```python
from build123d import *

# Parameters (mm, degrees)
BOSS_EXTRUDE1_DEPTH = 2.5
SKETCH2_R           = 1.2
CUT_EXTRUDE1_DEPTH  = 14.44432966


with BuildPart() as part:
    # Sketch1 → Boss-Extrude1 (new, symmetric)
    with BuildSketch(Plane.XY):
        with BuildLine():
            Line((5, 0), (11.5, 0))
            Line((11.5, 0), (11.5, -1.5))
            Line((11.5, -1.5), (6.32455532, -1.5))
            ThreePointArc((6.32455532, -1.5), (0, -6.5), (-6.32455532, -1.5))
            Line((-6.32455532, -1.5), (-11.5, -1.5))
            Line((-11.5, -1.5), (-11.5, 0))
            Line((-11.5, 0), (-5, 0))
            ThreePointArc((-5, 0), (0, -5), (5, 0))
        make_face()
    extrude(amount=BOSS_EXTRUDE1_DEPTH, both=True)

    # Sketch2 → Cut-Extrude1 (cut, through all)
    with BuildSketch(Plane(origin=(0, 0, 0), x_dir=(1, 0, 0), z_dir=(0, 1, 0))):
        with Locations(Location((-9, 0, 0), (0, 0, 270))):
            Circle(SKETCH2_R)
        with Locations(Location((9, 0, 0), (0, 0, 180))):
            Circle(SKETCH2_R)
    extrude(amount=-CUT_EXTRUDE1_DEPTH, mode=Mode.SUBTRACT)


solid = part.part
```
Design review of the part built by this model. Coordinates are the model's own, in mm. A direction names the side the tool comes from. Round coordinates to 2 decimals unless told otherwise and drop trailing zeros. Order: outer loops, then holes, each group sorted by start corner. A loop starts at its lowest first (then second) coordinate and runs counter-clockwise, first axis right, second up. Notation, with made-up numbers: (36, 10) - (61, 10) arc R23 ccw to (61, 32) - close; hole circle Ø6 at (42, -3.5). An arc over 180 degrees is marked (long way). Return JSON: item names as keys, results as strings.
Q1. Consider section D-D on y = -3.75. Write out the cut boundary in (x, z), plus the area to 3 significant figures.
Computed values:
{"outline": "(-5.31, -2.5) - (-3.31, -2.5) - (-3.31, 2.5) - (-5.31, 2.5) - close; (3.31, -2.5) - (5.31, -2.5) - (5.31, 2.5) - (3.31, 2.5) - close", "area": "20.0 mm2"}
Q2. For pin 1 Ø3 at (x, z) = (-2.5, 1.5) entering from +Y; pin 2 Ø2.5 at (x, z) = (-8, 1) entering from -Y, all flat-tipped, find the tip position at first contact; note any pin that passes through.
Computed values:
{"pin 1": "stops at y = -3", "pin 2": "stops at y = -1.5"}
Q3. Consider section C-C on z = 0. Write out the cut boundary in (x, y), plus the area to 3 significant figures.
Computed values:
{"outline": "(-11.5, -1.5) - (-10.2, -1.5) - (-10.2, 0) - (-11.5, 0) - close; (-7.8, -1.5) - (-6.32, -1.5) arc R6.5 ccw to (6.32, -1.5) - (7.8, -1.5) - (7.8, 0) - (5, 0) arc R5 cw to (-5, 0) - (-7.8, 0) - close; (10.2, -1.5) - (11.5, -1.5) - (11.5, 0) - (10.2, 0) - close", "area": "35.1 mm2"}
Q4. Consider section B-B on y = -1. Write out the cut boundary in (x, z), plus the area to 3 significant figures.
Computed values:
{"outline": "(-11.5, -2.5) - (-4.9, -2.5) - (-4.9, 2.5) - (-11.5, 2.5) - close; (4.9, -2.5) - (11.5, -2.5) - (11.5, 2.5) - (4.9, 2.5) - close; hole circle Ø2.4 at (-9, 0); hole circle Ø2.4 at (9, 0)", "area": "57.0 mm2"}
Q5. Consider section A-A on x = 9. Write out the cut boundary in (y, z).
Computed values:
{"outline": "(-1.5, -2.5) - (0, -2.5) - (0, -1.2) - (-1.5, -1.2) - close; (-1.5, 1.2) - (0, 1.2) - (0, 2.5) - (-1.5, 2.5) - close"}
Q6. The part is to be moulded in two halves that separate along X. For faces 1 (the flat face through (-11.5, -1, 0)), 2 (the cylindrical face through (0.1, -6.5, 0)), 3 (the cylindrical face through (0, -5, 0)), 4 (the flat face through (-0.8, -5.2, -2.5)), say which applies: pulls with the +X half, pulls with the -X half, needs draft (parallel to the pull), parting line crosses it, or undercut.
Computed values:
{"face 1": "pulls with the -X half", "face 2": "parting line crosses it", "face 3": "undercut", "face 4": "needs draft"}
Q7. Machinability: for faces 5 (the flat face through (-7.6, 0, 0)), 6 (the flat face through (-8, -1.5, 1)), 7 (the flat face through (8, -1.5, 1)), which of the approach directions +Z, -Z, +X, -X, +Y, -Y give a long, thin tool a straight path to every point of the face, cutting with its end or side? Answer none if there is none.
Computed values:
{"face 5": "+Z, -Z, +X, -X, +Y", "face 6": "+Z, -Z, -X, -Y", "face 7": "+Z, -Z, +X, -Y"}
Q8. Wall thickness on L1, parallel to Z at x = 9, y = -0.35; L2, parallel to Y at x = -9.5, z = -2; L3, parallel to X at y = -0.25, z = -2.1: over which ranges is each line inside the solid? List them lowest first. Write a range as [from, to].
Computed values:
{"L1": "z = [-2.5, -1.2], [1.2, 2.5]", "L2": "y = [-1.5, 0]", "L3": "x = [-11.5, -4.99], [4.99, 11.5]"}
